```python
from build123d import *

# Parameters (mm, degrees)
F0_W     = 153
F0_H     = 153
F1_DEPTH = 35
F3_D     = 12
F4_R     = 9
F5_R     = 2
F7_DEPTH = 3


with BuildPart() as f1:
    # F0 (on Top) → F1 (new body)
    with BuildSketch(Plane.XY):
        with Locations((76.5, 76.5)):
            Rectangle(F0_W, F0_H)
    extrude(amount=F1_DEPTH)

    # F3 (through all)
    with Locations(Plane.XY.offset(35)):
        with Locations((9, 144), (9, 129), (9, 114), (9, 99), (9, 84), (9, 69), (9, 54), (9, 39), (9, 24), (9, 9), (24, 9), (24, 24), (24, 39), (24, 54), (24, 69), (24, 84), (24, 99), (24, 114), (24, 129), (24, 144), (39, 144), (54, 144), (69, 144), (84, 144), (99, 144), (114, 144), (129, 144), (144, 144), (144, 129), (129, 129), (114, 129), (99, 129), (84, 129), (69, 129), (54, 129), (39, 129), (39, 114), (39, 99), (39, 84), (39, 69), (39, 54), (39, 39), (39, 24), (39, 9), (54, 9), (54, 24), (54, 39), (54, 54), (54, 69), (54, 84), (54, 99), (54, 114), (69, 114), (69, 99), (69, 84), (69, 69), (69, 54), (69, 39), (69, 24), (69, 9), (84, 9), (84, 24), (84, 39), (84, 54), (84, 69), (84, 84), (84, 99), (84, 114), (99, 114), (99, 99), (99, 84), (99, 69), (99, 54), (99, 39), (99, 24), (99, 9), (114, 9), (129, 9), (144, 9), (144, 24), (129, 24), (114, 24), (114, 39), (129, 39), (144, 39), (144, 54), (129, 54), (114, 54), (114, 69), (129, 69), (144, 69), (144, 84), (129, 84), (114, 84), (114, 99), (114, 114), (129, 114), (129, 99), (144, 99), (144, 114)):
            Hole(F3_D / 2)

    # F4
    f4_edges = [f1.edges().sort_by_distance(p)[0] for p in [
        (0, 153, 17.5),
        (0, 0, 17.5),
        (153, 0, 17.5),
        (153, 153, 17.5),
    ]]
    fillet(f4_edges, radius=F4_R)

    # F5
    f5_edges = [f1.edges().sort_by_distance(p)[0] for p in [
        (76.5, 0, 35),
        (150.363961, 2.636039, 35),
        (153, 76.5, 35),
    ]]
    fillet(f5_edges, radius=F5_R)

    # F6 (on face) → F7 (join)
    with BuildSketch(Plane(origin=(0, 0, 0), x_dir=(1, 0, 0), z_dir=(0, 0, -1))):
        with BuildLine():
            Line((144, 0), (9, 0))
            ThreePointArc((9, 0), (2.6360389693, -2.6360389693), (0, -9))
            Line((0, -9), (0, -144))
            ThreePointArc((0, -144), (2.6360389693, -150.3639610307), (9, -153))
            Line((9, -153), (144, -153))
            ThreePointArc((144, -153), (150.3639610307, -150.3639610307), (153, -144))
            Line((153, -144), (153, -9))
            ThreePointArc((153, -9), (150.3639610307, -2.6360389693), (144, 0))
        make_face()
    extrude(amount=-F7_DEPTH)


solid = f1.part
```
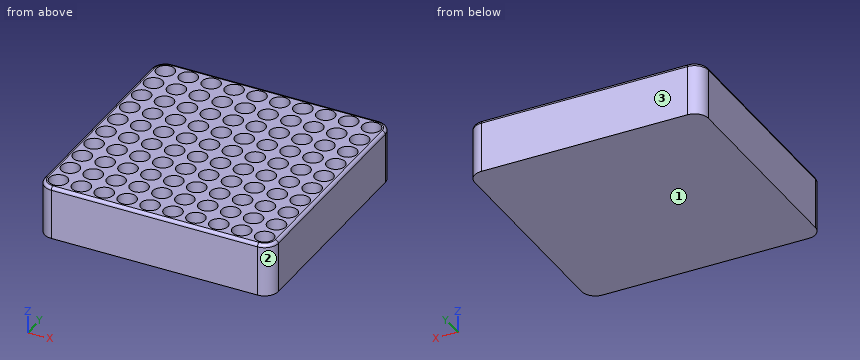
Part model, mm, in its own coordinate system. Face numbers are marked on the shaded views. Round coordinates to 2 decimals unless told otherwise and drop trailing zeros. Put each result on its own line as item: value. Start each with the question number.
1. Two-plate mould, pull along Y, no slides. Class the marked faces 1, 2 and 3: +Y half, -Y half, draft (parallel to the pull), parting line (faces both ways), or undercut.
2. Drill centre line: probe 1 along Z at (x, y) = (66.5, 140). Where is it in solid material? Low to high. Write a range as [from, to].
3. Drop flat-ended pins along their axis: pin 1 (13 mm diameter, centred on x = 69, y = 26, fed in from +Z); pin 2 (7 mm diameter, centred on x = 39, y = 114, fed in from +Z). Give the stop position or say it passes through.
4. Slice it at A-A on z = 16.5. State how many separate pieces and enclosed holes the cut face has, then the cut area to 3 significant figures.
Findings:
1. face 1: draft
1. face 2: -Y half
1. face 3: +Y half
2. probe 1: [0, 3]
3. pin 1: z = 35
3. pin 2: z = 3
4. separate pieces: 1
4. enclosed holes: 100
4. area: 12,000 mm2
